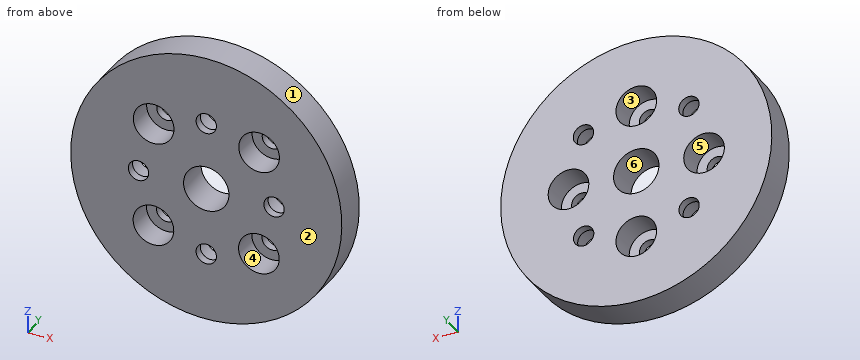
```python
from build123d import *

# Parameters (mm, degrees)
SKETCH2_R           = 20
BOSS_EXTRUDE1_DEPTH = 5
SKETCH3_R           = 3.35
CUT_EXTRUDE1_DEPTH  = 6
SKETCH4_R           = 1.5
CUT_EXTRUDE3_DEPTH  = 6
SKETCH6_R           = 3
CUT_EXTRUDE4_DEPTH  = 3.8
SKETCH7_R           = 1.5
CUT_EXTRUDE5_DEPTH  = 29.722813233
SKETCH8_R           = 3
CUT_EXTRUDE6_DEPTH  = 3.8


with BuildPart() as part:
    # Sketch2 → Boss-Extrude1 (new body)
    with BuildSketch(Plane(origin=(0, 0, 0), x_dir=(1, 0, 0), z_dir=(0, 1, 0))):
        with Locations(Location((0, 0, 0), (0, 0, 270))):
            Circle(SKETCH2_R)
    extrude(amount=BOSS_EXTRUDE1_DEPTH)

    # Sketch3 → Cut-Extrude1 (cut)
    with BuildSketch(Plane(origin=(0, 5, 0), x_dir=(1, 0, 0), z_dir=(0, 1, 0))):
        with Locations(Location((0, 0, 0), (0, 0, 270))):
            Circle(SKETCH3_R)
    extrude(amount=-CUT_EXTRUDE1_DEPTH, mode=Mode.SUBTRACT)

    # Sketch4 → Cut-Extrude3 (cut)
    with BuildSketch(Plane(origin=(0, 5, 0), x_dir=(1, 0, 0), z_dir=(0, 1, 0))):
        with Locations(Location((0, 10, 0), (0, 0, 270))):
            Circle(SKETCH4_R)
        with Locations(Location((10, 0, 0), (0, 0, 270))):
            Circle(SKETCH4_R)
        with Locations(Location((0, -10, 0), (0, 0, 270))):
            Circle(SKETCH4_R)
        with Locations(Location((-10, 0, 0), (0, 0, 270))):
            Circle(SKETCH4_R)
    extrude(amount=-CUT_EXTRUDE3_DEPTH, mode=Mode.SUBTRACT)

    # Sketch6 → Cut-Extrude4 (cut)
    with BuildSketch(Plane(origin=(0, 5, 0), x_dir=(1, 0, 0), z_dir=(0, 1, 0))):
        with Locations(Location((0, 10, 0), (0, 0, 270))):
            Circle(SKETCH6_R)
        with Locations(Location((10, 0, 0), (0, 0, 270))):
            Circle(SKETCH6_R)
        with Locations(Location((0, -10, 0), (0, 0, 270))):
            Circle(SKETCH6_R)
        with Locations(Location((-10, 0, 0), (0, 0, 270))):
            Circle(SKETCH6_R)
    extrude(amount=-CUT_EXTRUDE4_DEPTH, mode=Mode.SUBTRACT)

    # Sketch7 → Cut-Extrude5 (cut, through all)
    with BuildSketch(Plane.XZ):
        with Locations(Location((7.793746467, 7.762571482, 0), (0, 0, 270))):
            Circle(SKETCH7_R)
        with Locations(Location((7.762571482, -7.793746467, 0), (0, 0, 270))):
            Circle(SKETCH7_R)
        with Locations(Location((-7.793746467, -7.762571482, 0), (0, 0, 270))):
            Circle(SKETCH7_R)
        with Locations(Location((-7.762571482, 7.793746467, 0), (0, 0, 270))):
            Circle(SKETCH7_R)
    extrude(amount=-CUT_EXTRUDE5_DEPTH, mode=Mode.SUBTRACT)

    # Sketch8 → Cut-Extrude6 (cut)
    with BuildSketch(Plane(origin=(0, 0, 0), x_dir=(-1, 0, 0), z_dir=(0, -1, 0))):
        with Locations(Location((-7.793746467, -7.762571482, 0), (0, 0, 90))):
            Circle(SKETCH8_R)
        with Locations(Location((-7.762571482, 7.793746467, 0), (0, 0, 90))):
            Circle(SKETCH8_R)
        with Locations(Location((7.793746467, 7.762571482, 0), (0, 0, 90))):
            Circle(SKETCH8_R)
        with Locations(Location((7.762571482, -7.793746467, 0), (0, 0, 90))):
            Circle(SKETCH8_R)
    extrude(amount=-CUT_EXTRUDE6_DEPTH, mode=Mode.SUBTRACT)


solid = part.part
```
For this review, take the finished solid that the model builds, in its own axes (mm). Face numbers are marked on the shaded views. A direction names the side the tool comes from. Round coordinates to 2 decimals unless told otherwise and drop trailing zeros. Loops run counter-clockwise (first coordinate to the right, second up) from the corner with the lowest first, then second, coordinate; pieces in that order, holes last.
Q1. Add section D-D on x = 10. Write out the cut boundary in (y, z).
Result sheet:
outline: (0, -17.32) - (5, -17.32) - (5, -3) - (1.2, -3) - (1.2, -1.5) - (0, -1.5) - (0, -5.8) - (3.8, -5.8) - (3.8, -9.79) - (0, -9.79) - close; (0, 1.5) - (1.2, 1.5) - (1.2, 3) - (5, 3) - (5, 17.32) - (0, 17.32) - (0, 9.8) - (3.8, 9.8) - (3.8, 5.73) - (0, 5.73) - close
Q2. Mouldability with a two-part tool opening along X and no side actions: class the marked faces 1, 2 and 3 as +X half, -X half, draft (parallel to the pull), parting line (faces both ways), or undercut.
Result sheet:
face 1: parting line
face 2: draft
face 3: undercut
Q3. Add section C-C on y = 0.55. Give the number of separate pieces and of enclosed holes in the cut face, plus the area to 3 significant figures.
Result sheet:
separate pieces: 1
enclosed holes: 9
area: 1,080 mm2
Q4. To check wall thickness, follow line 1 along X through (y, z) = (0.75, 0); line 2 along X through (y, z) = (0.8, -1); line 3 along Z through (x, y) = (6.5, 3). State the ranges of each line that lie inside material, in increasing order.
Result sheet:
line 1: x = -20 to -11.5, -8.5 to -3.35, 3.35 to 8.5, 11.5 to 20
line 2: x = -19.97 to -11.12, -8.88 to -3.2, 3.2 to 8.88, 11.12 to 19.97
line 3: z = -18.91 to -10.52, -5.07 to 5.06, 10.47 to 18.91
Q5. Add section B-B on x = 0. Write out the cut boundary in (y, z), plus the area to 3 significant figures.
Result sheet:
outline: (0, -20) - (5, -20) - (5, -13) - (1.2, -13) - (1.2, -11.5) - (0, -11.5) - close; (0, -8.5) - (1.2, -8.5) - (1.2, -7) - (5, -7) - (5, -3.35) - (0, -3.35) - close; (0, 3.35) - (5, 3.35) - (5, 7) - (1.2, 7) - (1.2, 8.5) - (0, 8.5) - close; (0, 11.5) - (1.2, 11.5) - (1.2, 13) - (5, 13) - (5, 20) - (0, 20) - close
area: 114 mm2
Q6. Add section A-A on z = 0. Write out the cut boundary in (x, y), plus the area to 3 significant figures.
Result sheet:
outline: (-20, 0) - (-11.5, 0) - (-11.5, 1.2) - (-13, 1.2) - (-13, 5) - (-20, 5) - close; (-8.5, 0) - (-3.35, 0) - (-3.35, 5) - (-7, 5) - (-7, 1.2) - (-8.5, 1.2) - close; (3.35, 0) - (8.5, 0) - (8.5, 1.2) - (7, 1.2) - (7, 5) - (3.35, 5) - close; (11.5, 0) - (20, 0) - (20, 5) - (13, 5) - (13, 1.2) - (11.5, 1.2) - close
area: 114 mm2
Q7. Insertion check: pin 1 Ø3 at (x, z) = (-0.5, 10.5) entering from +Y; pin 2 Ø2.5 at (x, z) = (10, 0) entering from -Y; pin 3 Ø3 at (y, z) = (0.5, 14.5) entering from -X; pin 4 Ø1.5 at (y, z) = (0.5, -0.5) entering from -X. Each pin has a flat end and moves straight along its axis. Give the tip position at first contact, or say it passes through.
Result sheet:
pin 1: stops at y = 1.2
pin 2: passes through
pin 3: stops at x = -15.2
pin 4: stops at x = -20
Q8. Machinability: for the marked faces 4, 5 and 6, which of the approach directions +Z, -Z, +X, -X, +Y, -Y give a long, thin tool a straight path to every point of the face, cutting with its end or side? Answer none if there is none.
Result sheet:
face 4: -Y
face 5: +Y
face 6: +Y, -Y
